```python
from build123d import *

# Parameters (mm, degrees)
SKETCH1_W           = 12.7
SKETCH1_H           = 22.86
SKETCH1_R           = 1.75
BOSS_EXTRUDE1_DEPTH = 3.81
SKETCH2_W           = 12.7
SKETCH2_H           = 7.62
CUT_EXTRUDE1_DEPTH  = 0.889


with BuildPart() as part:
    # Sketch1 → Boss-Extrude1 (new body)
    with BuildSketch(Plane.XY):
        Rectangle(SKETCH1_W, SKETCH1_H)
        with Locations(Location((0, 7.62, 0), (0, 0, 180))):
            Circle(SKETCH1_R, mode=Mode.SUBTRACT)
        with Locations(Location((0, -7.62, 0), (0, 0, 180))):
            Circle(SKETCH1_R, mode=Mode.SUBTRACT)
    extrude(amount=BOSS_EXTRUDE1_DEPTH)

    # Sketch2 → Cut-Extrude1 (cut)
    with BuildSketch(Plane.XY.offset(3.81)):
        Rectangle(SKETCH2_W, SKETCH2_H)
    extrude(amount=-CUT_EXTRUDE1_DEPTH, mode=Mode.SUBTRACT)


solid = part.part
```
Geometry check sheet. Reference: the model listing, model coordinates, mm. A direction names the side the tool comes from. Round coordinates to 2 decimals unless told otherwise and drop trailing zeros. Loops run counter-clockwise (first coordinate to the right, second up) from the corner with the lowest first, then second, coordinate; pieces in that order, holes last. Notation, with made-up numbers: (16.25, 18) - (51.25, 18) arc R18 ccw to (51.25, 29) - close; hole circle Ø8 at (30, -5.5). An arc over 180 degrees is marked (long way). Write each question's results on one line, items separated by ' | '. Start each with the question number.
Q1. Thickness scan on line 1 (Y direction, x = 0, z = 2.65); line 2 (X direction, y = -7.62, z = 2.15); line 3 (Y direction, x = 1, z = 0.95). Record the ranges inside material, lowest first. Write a range as [from, to].
Q2. Cross-section at D-D on x = -2.5. Enter the section's corners in (y, z), and give its area (3 significant figures).
Q3. Access from +Z, -Z, +X, -X, +Y, -Y to the whole of each face (thin tool, end or side, straight path). Record for faces 1 (the cylindrical face through (0.38, -5.91, 1.88)), 2 (the flat face through (-0.1, 3.81, 3.4)).
Q4. Cross-section at B-B on x = 0. Enter the section's corners in (y, z), and give its area (3 significant figures).
Q5. Cross-section at C-C on z = 2.35. Enter the section's corners in (x, y).
Q6. Cross-section at A-A on y = -7.62. Enter the section's corners in (x, z), and give its area (3 significant figures).
Q7. Gauge pin test, flat ends, axial feed: P1, Ø3, axis at x = 0, y = -7.62, coming from the -Z side; P2, Ø2.5, axis at x = 0, y = 1, coming from the +Z side. Record the tip position at first contact, or that the pin passes through.
Answers below:
1) line 1: y = [-11.43, -9.37], [-5.87, 5.87], [9.37, 11.43] | line 2: x = [-6.35, -1.75], [1.75, 6.35] | line 3: y = [-11.43, -9.06], [-6.18, 6.18], [9.06, 11.43]
2) outline: (-11.43, 0) - (11.43, 0) - (11.43, 3.81) - (3.81, 3.81) - (3.81, 2.92) - (-3.81, 2.92) - (-3.81, 3.81) - (-11.43, 3.81) - close | area: 80.3 mm²
3) face 1: +Z, -Z | face 2: +Z, +X, -X
4) outline: (-11.43, 0) - (-9.37, 0) - (-9.37, 3.81) - (-11.43, 3.81) - close; (-5.87, 0) - (5.87, 0) - (5.87, 3.81) - (3.81, 3.81) - (3.81, 2.92) - (-3.81, 2.92) - (-3.81, 3.81) - (-5.87, 3.81) - close; (9.37, 0) - (11.43, 0) - (11.43, 3.81) - (9.37, 3.81) - close | area: 53.7 mm²
5) outline: (-6.35, -11.43) - (6.35, -11.43) - (6.35, 11.43) - (-6.35, 11.43) - close; hole circle Ø3.5 at (0, -7.62); hole circle Ø3.5 at (0, 7.62)
6) outline: (-6.35, 0) - (-1.75, 0) - (-1.75, 3.81) - (-6.35, 3.81) - close; (1.75, 0) - (6.35, 0) - (6.35, 3.81) - (1.75, 3.81) - close | area: 35.1 mm²
7) P1: passes through | P2: stops at z = 2.92
